Here's how the part is built. I have some questions about the finished solid (model axes, mm). A direction names the side the tool comes from. Coordinates: 2 decimals unless noted, no trailing zeros. Write each loop counter-clockwise with the first axis right and the second up, starting at its lowest first coordinate (ties: lowest second). Pieces come first, ordered by that corner, then holes.
Item 1: I want a section at B-B (y = 0). Count the separate pieces of the cut face and the enclosed holes in it, and give its area (3 significant figures).
Item 2: If we mould it in two halves opening along X, with no side actions, what happens to faces 5 (the face through (155.575, -10, 0)), 6 (the face through (-14.274, 0.628, 0.278)), 7 (the face through (40, 0, 19.837))? For each: pulls with the +X half, pulls with the -X half, needs draft (parallel to the pull), parting line crosses it, or undercut.
Item 3: I'm going to push flat-ended pins straight in: P1, Ø20.5, axis at x = 168.275, z = 0, coming from the +Y side; P2, Ø1.5, axis at x = 89.5, y = 20.5, coming from the +Z side; P3, Ø10, axis at x = 75.5, z = -14.5, coming from the +Y side. Where does each tip first touch, or does it pass through?
Item 4: Please list where these lines run through material, in increasing order: line 1 (X direction, y = -2, z = 0) (3 decimals); line 2 (X direction, y = 4, z = 0) (3 decimals); line 3 (Y direction, x = 170.5, z = -13).
Item 5: I want a section at A-A (z = 0). Please give me the cut outline in (x, y) (1 decimal).
Item 6: For faces 1 (the face through (149.57, -4.77, 15.14)), 2 (the face through (168, 7.137, 7)), 3 (the face through (57.463, 26.986, -0.312)), 4 (the face through (57.463, -26.986, 0.312)), which set-ups out of +Z, -Z, +X, -X, +Y, -Y let a thin tool reach every point of the face, with its end or its side?
Item 7: I want a section at D-D (x = 60). Please give me the cut outline in (y, z) (1 decimal).
Item 8: I want a section at C-C (x = 4). Please give me the cut outline in (y, z), and give its area (3 significant figures).
from build123d import *

# Parameters (mm, degrees)
CORTAR_EXTRUIR1_DEPTH      = 226.603802328
CORTAR_EXTRUIR1_DEPTH_BACK = 226.603802328
CORTAR_EXTRUIR2_START      = -25.4
CORTAR_EXTRUIR2_DEPTH      = 25.4
CORTAR_EXTRUIR3_REACH      = 189.595
CROQUIS5_R                 = 6.35
CORTAR_EXTRUIR4_REACH      = 191.15
CROQUIS6_R                 = 14.2875


with BuildPart() as part:
    # Croquis2 → Revolución1 (revolve)
    with BuildSketch(Plane.XY, mode=Mode.PRIVATE) as revoluci_n1_sk:
        with BuildLine():
            Line((-38.1, 0), (180.975, 0))
            Line((180.975, 0), (180.975, 15.875))
            Line((180.975, 15.875), (130.175, 15.875))
            Line((130.175, 15.875), (88.9, 26.9875))
            Line((88.9, 26.9875), (26.893955524, 26.9875))
            ThreePointArc((26.893955524, 26.9875), (-14.610788728, 35.187140446), (-38.1, 0))
        make_face()
    revolve(revoluci_n1_sk.sketch.rotate(Axis((-38.1, 0, 0), (1, 0, 0)), 90), axis=Axis((-38.1, 0, 0), (1, 0, 0)))

    # Croquis3 → Cortar-Extruir1 (cut, two sides: drawn at the far end of the back side and taken through both)
    with BuildSketch(Plane(origin=(180.975, 0, 0), x_dir=(0, 0, -1), z_dir=(1, 0, 0)).offset(-CORTAR_EXTRUIR1_DEPTH_BACK)):
        with BuildLine():
            Line((-19.8374, 32.528257888), (-19.8374, -32.528257888))
            ThreePointArc((-19.8374, -32.528257888), (-38.1, 0), (-19.8374, 32.528257888))
        make_face()
        with BuildLine():
            Line((19.8374, 32.528257888), (19.8374, -32.528257888))
            ThreePointArc((19.8374, -32.528257888), (38.1, 0), (19.8374, 32.528257888))
        make_face()
    extrude(amount=CORTAR_EXTRUIR1_DEPTH + CORTAR_EXTRUIR1_DEPTH_BACK, mode=Mode.SUBTRACT)

    # Croquis4 → Cortar-Extruir2 (cut)
    with BuildSketch(Plane(origin=(180.975, 0, 0), x_dir=(0, 0, -1), z_dir=(1, 0, 0)).offset(CORTAR_EXTRUIR2_START)):
        with BuildLine():
            Line((-14.180026313, 7.1374), (14.180026313, 7.1374))
            ThreePointArc((14.180026313, 7.1374), (0, 15.875), (-14.180026313, 7.1374))
        make_face()
        with BuildLine():
            Line((-14.180026313, -7.1374), (14.180026313, -7.1374))
            ThreePointArc((14.180026313, -7.1374), (0, -15.875), (-14.180026313, -7.1374))
        make_face()
    extrude(amount=CORTAR_EXTRUIR2_DEPTH, mode=Mode.SUBTRACT)

    # Croquis5 → Cortar-Extruir3 (cut, up to next)
    with BuildSketch(Plane(origin=(0, 7.1374, 0), x_dir=(1, 0, 0), z_dir=(0, 1, 0)), mode=Mode.PRIVATE) as cortar_extruir3_sk1:
        with Locations(Location((168.275, 0, 0), (0, 0, 270))):
            Circle(CROQUIS5_R)
    cortar_extruir3_tool1 = extrude(cortar_extruir3_sk1.sketch, amount=-CORTAR_EXTRUIR3_REACH, mode=Mode.PRIVATE) & part.part
    add(cortar_extruir3_tool1.solids().sort_by_distance((168.275, 7.1374, 0))[0], mode=Mode.SUBTRACT)

    # Croquis6 → Cortar-Extruir4 (cut, up to next)
    with BuildSketch(Plane.XY.offset(19.8374), mode=Mode.PRIVATE) as cortar_extruir4_sk1:
        Circle(CROQUIS6_R)
    cortar_extruir4_tool1 = extrude(cortar_extruir4_sk1.sketch, amount=-CORTAR_EXTRUIR4_REACH, mode=Mode.PRIVATE) & part.part
    add(cortar_extruir4_tool1.solids().sort_by_distance((0, 0, 19.8374))[0], mode=Mode.SUBTRACT)


solid = part.part
Answer:
1. separate pieces: 2
1. enclosed holes: 1
1. area: 6,900 mm2
2. face 5: pulls with the +X half
2. face 6: undercut
2. face 7: needs draft
3. P1: stops at y = 7.14
3. P2: stops at z = 18.21
3. P3: stops at y = 25.26
4. line 1: x = -38.047 to -14.147, 14.147 to 161.925, 174.625 to 180.975
4. line 2: x = -37.889 to -13.716, 13.716 to 161.925, 174.625 to 180.975
4. line 3: y = -7.14 to 7.14
5. outline: (26.9, -27) - (88.9, -27) - (130.2, -15.9) - (155.6, -15.9) - (155.6, -7.1) - (161.9, -7.1) - (161.9, 7.1) - (155.6, 7.1) - (155.6, 15.9) - (130.2, 15.9) - (88.9, 27) - (26.9, 27) arc R38.1 ccw (long way) to start; (174.6, -7.1) - (181, -7.1) - (181, 7.1) - (174.6, 7.1) - close; hole circle Ø28.6 at (0, 0)
6. face 1: +X
6. face 2: +Z, -Z, +X, +Y
6. face 3: +X, +Y
6. face 4: +X, -Y
7. outline: (-18.3, -19.8) - (18.3, -19.8) arc R27 ccw to (18.3, 19.8) - (-18.3, 19.8) arc R27 ccw to start
8. outline: (-32.28, -19.84) - (-13.72, -19.84) - (-13.72, 19.84) - (-32.28, 19.84) arc R37.89 ccw to start; (13.72, -19.84) - (32.28, -19.84) arc R37.89 ccw to (32.28, 19.84) - (13.72, 19.84) - close
8. area: 1,770 mm2
